Work out the finished part from the listing and answer in its coordinate system (mm). Face numbers are marked on the shaded views. A direction names the side the tool comes from. Give positions to 0.01 mm unless a question says otherwise; leave off trailing zeros. Loops run counter-clockwise (first coordinate to the right, second up) from the corner with the lowest first, then second, coordinate; pieces in that order, holes last.
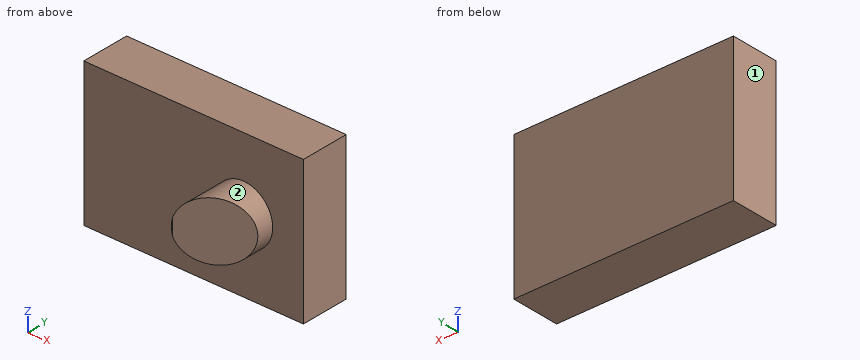
from build123d import *

# Parameters (mm, degrees)
F0_W     = 114.426647
F0_H     = 74.959393
F1_DEPTH = 25.4
F2_R     = 15.240971
F3_DEPTH = 25.4
F5_DEPTH = 25.4


with BuildPart() as f1:
    # F0 (on Front) → F1 (new body)
    with BuildSketch(Plane.XZ):
        with Locations((4.968898, -0.141972)):
            Rectangle(F0_W, F0_H)
    extrude(amount=F1_DEPTH)

    # F2 (on face) → F3 (join)
    with BuildSketch(Plane.XZ.offset(25.4)):
        with Locations((30.949144, 0)):
            Circle(F2_R)
    extrude(amount=F3_DEPTH)

    # F4 (on Top) → F5 (cut, symmetric)
    with BuildSketch(Plane.XY):
        Polygon((50.745651, -52.68006), (46.725634, -33.919994), (12.957521, -52.68006), align=None)
    extrude(amount=F5_DEPTH, both=True, mode=Mode.SUBTRACT)


solid = f1.part
Item 1: Find section B-B, the plane x = 24.5. Write down the section's boundary in (y, z), plus the area to 3 significant figures.
Item 2: Find section C-C, the plane y = -29. Write down the section's boundary in (x, z), plus the area to 3 significant figures.
Item 3: Find section A-A, the plane z = 0. Write down the section's boundary in (x, y).
Item 4: Consider line 1 (Y direction, x = -13, z = 20); line 2 (Y direction, x = 39, z = 0.5); line 3 (X direction, y = -41, z = -11). Determine where each line is inside the solid, lowest interval first.
Item 5: Flat-ended cylindrical pins translate along their axes: pin 1 Ø2 at (y, z) = (-29, 14) entering from +X; pin 2 Ø6 at (x, z) = (7.5, -3.5) entering from -Y. Find the tip coordinate at first contact, or state that the pin passes through.
Item 6: For the marked faces 1 and 2, determine the directions among +Z, -Z, +X, -X, +Y, -Y from which every point of the face is accessible in a straight line to the end or side of a thin tool.
Item 7: Find section D-D, the plane x = 10.5. Write down the section's boundary in (y, z), plus the area to 3 significant figures.
Ans:
1. outline: (-46.27, -13.81) - (-25.4, -13.81) - (-25.4, -37.62) - (0, -37.62) - (0, 37.34) - (-25.4, 37.34) - (-25.4, 13.81) - (-46.27, 13.81) - close
1. area: 2,480 mm2
2. outline: circle Ø30.48 at (30.95, 0)
2. area: 730 mm2
3. outline: (-52.24, -25.4) - (15.71, -25.4) - (15.71, -50.8) - (16.34, -50.8) - (46.19, -34.22) - (46.19, -25.4) - (62.18, -25.4) - (62.18, 0) - (-52.24, 0) - close
4. line 1: y = -25.4 to 0
4. line 2: y = -38.21 to 0
4. line 3: x = 20.4 to 33.98
5. pin 1: stops at x = 38.9
5. pin 2: stops at y = -25.4
6. face 1: +Z, -Z, -X, +Y, -Y
6. face 2: -Y
7. outline: (-25.4, -37.62) - (0, -37.62) - (0, 37.34) - (-25.4, 37.34) - close
7. area: 1,900 mm2
